```python
from build123d import *

# Parameters (mm, degrees)
P_IDAT_VYSUNUT_M1_DEPTH  = 8
ODEBRAT_VYSUNUT_M1_DEPTH = 165.210299616
SKICA3_W                 = 2
SKICA3_H                 = 2
P_IDAT_VYSUNUT_M2_DEPTH  = 4
SKICA5_W                 = 16
SKICA5_H                 = 8
P_IDAT_VYSUNUT_M3_DEPTH  = 8
ODEBRAT_VYSUNUT_M4_DEPTH = 165.210299616
SKICA4_W                 = 2.4
SKICA4_H                 = 2.4
ODEBRAT_VYSUNUT_M2_DEPTH = 4.4
ODEBRAT_VYSUNUT_M5_DEPTH = 165.210299616
ODEBRAT_VYSUNUT_M6_DEPTH = 165.210299616
ZAOBLIT1_R               = 150


with BuildPart() as part:
    # Skica1 → Přidat vysunutím1 (new body)
    with BuildSketch(Plane(origin=(0, 0, 0), x_dir=(1, 0, 0), z_dir=(0, 1, 0))):
        Polygon((0, 0), (0, -66), (150.15, -32.97), (150.15, 0), (142.85, 0), (142.85, -26.8965309), (7.3, -56.714822608), (7.3, 0), align=None)
    extrude(amount=P_IDAT_VYSUNUT_M1_DEPTH)

    # Skica2 → Odebrat vysunutím1 (cut, through all)
    with BuildSketch(Plane(origin=(0, 8, 0), x_dir=(1, 0, 0), z_dir=(0, 1, 0))):
        Polygon((0, -50.6), (1, -50.6), (3.2, -48.6), (3.2, -55), (1, -53), (0, -53), align=None)
    extrude(amount=-ODEBRAT_VYSUNUT_M1_DEPTH, mode=Mode.SUBTRACT)

    # Skica3 → Přidat vysunutím2 (add)
    with BuildSketch(Plane.ZY):
        with Locations((11.3, 4)):
            Rectangle(SKICA3_W, SKICA3_H)
        with Locations((39.1, 4)):
            Rectangle(SKICA3_W, SKICA3_H)
    extrude(amount=P_IDAT_VYSUNUT_M2_DEPTH)

    # Skica5 → Přidat vysunutím3 (add)
    with BuildSketch(Plane(origin=(0, 8, 0), x_dir=(1, 0, 0), z_dir=(0, 1, 0))):
        with Locations((8, -9)):
            Rectangle(SKICA5_W, SKICA5_H)
        with Locations((142.15, -9)):
            Rectangle(SKICA5_W, SKICA5_H)
    extrude(amount=-P_IDAT_VYSUNUT_M3_DEPTH)

    # Skica7 → Odebrat vysunutím4 (cut, through all)
    with BuildSketch(Plane.XZ):
        Polygon((7.3, 13), (16, 5), (16, 13), align=None)
        Polygon((134.15, 5), (134.15, 13), (142.85, 13), align=None)
    extrude(amount=-ODEBRAT_VYSUNUT_M4_DEPTH, mode=Mode.SUBTRACT)

    # Skica4 → Odebrat vysunutím2 (cut)
    with BuildSketch(Plane(origin=(150.15, 0, 0), x_dir=(0, 0, -1), z_dir=(1, 0, 0))):
        with Locations((-19.2, 4)):
            Rectangle(SKICA4_W, SKICA4_H)
        with Locations((-6.4, 4)):
            Rectangle(SKICA4_W, SKICA4_H)
    extrude(amount=-ODEBRAT_VYSUNUT_M2_DEPTH, mode=Mode.SUBTRACT)

    # Skica8 → Odebrat vysunutím5 (cut, through all)
    with BuildSketch(Plane(origin=(0, 8, 0), x_dir=(1, 0, 0), z_dir=(0, 1, 0))):
        Polygon((150.15, -24.5), (149.15, -24.5), (146.95, -22.5), (146.95, -28.9), (149.15, -26.9), (150.15, -26.9), align=None)
    extrude(amount=-ODEBRAT_VYSUNUT_M5_DEPTH, mode=Mode.SUBTRACT)

    # Skica9 → Odebrat vysunutím6 (cut, through all)
    with BuildSketch(Plane(origin=(0, 8, 0), x_dir=(1, 0, 0), z_dir=(0, 1, 0))):
        Polygon((0, -61), (22.729336966, -61), (0, -66), align=None)
    extrude(amount=-ODEBRAT_VYSUNUT_M6_DEPTH, mode=Mode.SUBTRACT)

    # Zaoblit1
    zaoblit1_edges = [part.edges().sort_by_distance(p)[0] for p in [
        (22.729336966, 4, 61),
    ]]
    fillet(zaoblit1_edges, radius=ZAOBLIT1_R)


solid = part.part
```
Model file for the job. Use its own axes, mm. A direction names the side the tool comes from. Give positions to 0.01 mm unless a question says otherwise; leave off trailing zeros. Loops run counter-clockwise (first coordinate to the right, second up) from the corner with the lowest first, then second, coordinate; pieces in that order, holes last. Notation, with made-up numbers: (78, 13) - (103, 13) arc R16 cw to (103, 23) - close; hole circle Ø9 at (13, 64). An arc over 180 degrees is marked (long way). One line per item, written item: value. Start each with the question number.
1. Probe L1, parallel to X at y = 3.75, z = 26; L2, parallel to X at y = 6, z = 19.5; L3, parallel to Z at x = 88, y = 7.5. List the from-to ranges inside material, lowest first. Write a range as from..to.
2. Slice it at D-D (x = 35.5). List the corners of the cut face in (y, z).
3. Which spindle directions (+Z, -Z, +X, -X, +Y, -Y) get a long thin tool onto all of the face, cutting with end or side? Do faces 5 (the flat face through (142.85, 4, 2)), 6 (the flat face through (0, 4, 57)), 7 (the flat face through (7.3, 4, 35)), 8 (the flat face through (150.15, 4, 12)). Say none if no direction does.
4. Slice it at C-C (x = 54). List the corners of the cut face in (y, z), plus the area to 3 significant figures.
5. Slice it at A-A (z = 43.5). List the corners of the cut face in (x, y), plus the area to 3 significant figures.
6. Pin check, flat tips, straight feed: pin 1 (1 mm diameter, centred on x = -2.5, z = 11.5, fed in from +Y); pin 2 (1.5 mm diameter, centred on x = 34, y = 2, fed in from -Z); pin 3 (2 mm diameter, centred on x = 91.5, y = 5.5, fed in from -Z); pin 4 (1.9 mm diameter, centred on y = 3.5, z = 19.5, fed in from +X). Stop position of each tip, or through.
7. Pull direction Z, two halves, no side cores. Call faces 1 (the flat face through (3.2, 4, 52)), 2 (the cylindrical face through (22.86, 3.944, 60.097)), 3 (the flat face through (138.561, 3.944, 9.056)), 4 (the flat face through (150.15, 4, 30)): pulls with the +Z half, pulls with the -Z half, needs draft (parallel to the pull), parting line crosses it, or undercut.
8. Slice it at B-B (y = 6.5). List the corners of the cut face in (x, z), plus the area to 3 significant figures.
Solution:
1. L1: x = 0..7.3, 142.85..146.95
1. L2: x = 0..7.3, 142.85..150.15
1. L3: z = 38.96..46.64
2. outline: (0, 50.51) - (8, 50.51) - (8, 58.16) - (0, 58.16) - close
3. face 5: -Z, +Y, -Y
3. face 6: +Z, -X, +Y, -Y
3. face 7: +Y, -Y
3. face 8: +Z, -Z, +X, +Y, -Y
4. outline: (0, 46.44) - (8, 46.44) - (8, 54.12) - (0, 54.12) - close
4. area: 61.4 mm^2
5. outline: (0, 0) - (7.3, 0) - (7.3, 8) - (0, 8) - close; (67.37, 0) - (102.28, 0) - (102.28, 8) - (67.37, 8) - close
5. area: 338 mm^2
6. pin 1: stops at y = 5
6. pin 2: stops at z = 50.68
6. pin 3: stops at z = 37.97
6. pin 4: stops at x = 150.15
7. face 1: undercut
7. face 2: pulls with the +Z half
7. face 3: undercut
7. face 4: needs draft
8. outline: (0, 0) - (7.3, 0) - (7.3, 5) - (16, 5) - (7.3, 13) - (7.3, 56.71) - (142.85, 26.9) - (142.85, 13) - (134.15, 5) - (142.85, 5) - (142.85, 0) - (150.15, 0) - (150.15, 24.5) - (149.15, 24.5) - (146.95, 22.5) - (146.95, 28.9) - (149.15, 26.9) - (150.15, 26.9) - (150.15, 32.97) - (38.65, 57.5) arc R150 ccw to (6.43, 61) - (0, 61) - (0, 53) - (1, 53) - (3.2, 55) - (3.2, 48.6) - (1, 50.6) - (0, 50.6) - close
8. area: 1,740 mm^2
